Autodesk Inventor part; units mm, degrees
ref_plane "Work Plane2" through (0, 1, 0) normal (0, -1, 0) x (1, 0, 0)
ref_plane "YZ Plane" through (0, 0, 0) normal (1, 0, 0) x (0, 1, 0)
ref_plane "XZ Plane" through (0, 0, 0) normal (0, 1, 0) x (-1, 0, 0)
sketch "Sketch1" plane through (0, 0, 0) normal (0, 1, 0) x (-1, 0, 0)
  line L0 (0, 0) -> (20, 0)
  line L1 (20, 0) -> (20, -2)
  line L2 (20, -2) -> (0, -2)
  line L3 (0, -2) -> (0, 0)
  dimension "d0" = 20
  dimension "d1" = 2
extrude "Extrusion1" add sketch "Sketch1" along normal blind 2
sketch "Sketch2" plane through (0, 2, 0) normal (0, 1, 0) x (1, 0, 0)
  line L0 (0, 2) -> (-20, 2)
  line L1 (0, 2) -> (0, 4)
  line L2 (0, 4) -> (2, 4)
  line L3 (2, 4) -> (2, -2)
  line L4 (2, -2) -> (0, -2)
  line L5 (0, 0) -> (0, 2)
  line L6 (0, -2) -> (0, 0)
  dimension "d4" = 2
  dimension "d5" = 2
  dimension "d6" = 6
extrude "Extrusion2" add sketch "Sketch2" against normal blind 2
sketch "Sketch3" plane through (0, 2, 0) normal (0, 1, 0) x (1, 0, 0)
  line L0 (0, 0) -> (0, -2)
  line L1 (0, -2) -> (0, -1)
  line L2 (2, 4) -> (2, -2)
  line L3 (2, -2) -> (2, -0.5)
  line L4 (2, -0.5) -> (1, -0.5)
  circle A0 centre (1, -0.5) radius 0.5
  line L5 (2, 1) -> (1.5, 1)
  circle A1 centre (1, 2.5) radius 0.5
  dimension "d9" = 1.5
  dimension "d10" = 1
  dimension "d11" = 1
extrude "Extrusion3" cut sketch "Sketch3" against normal blind 2
sketch "Sketch4" plane through (0, 2, -4) normal (-1, 0, 0) x (0, 0, 1)
  line L0 (2, 0) -> (4, 0)
  line L1 (3, 0) -> (3, -2)
  line L2 (2, -2) -> (4, -2)
  circle A0 centre (3, -1) radius 1
  line L3 (2, -2) -> (2, 0)
  circle A1 centre (3, -1) radius 1.4142
extrude "Extrusion4" cut sketch "Sketch4" along normal blind 100 contours L0 A0 L3 | L3 A1 | L0 A1 L2 A0 | A0 L2 L3
ref_plane "Work Plane1" through (-14, 1, -1) normal (-1, 0, 0) x (0, 0, 1)
sketch "Sketch5" plane through (-14, 1, -1) normal (-1, 0, 0) x (0, 0, 1)
  circle A0 centre (0, 0) radius 5
  point P0 (1, -1)
  dimension "d17" = 10
extrude "Extrusion5" add sketch "Sketch5" along normal mid plane 1
sketch "Sketch6" plane through (-20, 1, -1) normal (-1, 0, 0) x (0, 0, 1)
  circle A0 centre (0, 0) radius 5
  point P0 (1, -1)
extrude "Extrusion6" cut sketch "Sketch6" against normal blind 5.5
sketch "Sketch7" plane through (-13.5, 1, -1) normal (1, 0, 0) x (0, 0, -1)
  circle A0 centre (0, 0) radius 5
  circle A1 centre (0, 0) radius 5
  point P0 (-1, -1)
extrude "Extrusion7" add sketch "Sketch7" along normal blind 13.5
sketch "Sketch8" plane through (0, 0, 0) normal (0, -1, 0) x (1, 0, 0)
  line L0 (2, -4) -> (-1, -4)
  line L1 (-1, -4) -> (-1, -6.7389)
  line L2 (-1, -6.7389) -> (2, -6.7389)
  line L3 (2, -6.7389) -> (2, -4)
  line L4 (2, -4) -> (2, 2)
  line L5 (2, 2) -> (-1, 2)
  line L6 (-1, 2) -> (-1, 5.2785)
  line L7 (-1, 5.2785) -> (2, 5.2785)
  line L8 (2, 5.2785) -> (2, 2)
  line L9 (2, 5.2785) -> (-1, 5.2785)
  line L10 (-1, 5.2785) -> (-1, -6.7389)
  line L11 (-1, -6.7389) -> (2, -6.7389)
  line L12 (2, -6.7389) -> (2, 5.2785)
  point P0 (0, 0)
  dimension "d24" = 3
  dimension "d25" = 3
extrude "Extrusion8" cut sketch "Sketch8" along normal blind 13.5
ref_plane "Work Plane2" through (0, 1, 0) normal (0, -1, 0) x (1, 0, 0)
mirror "Mirror1" about plane through (0, 1, 0) normal (0, -1, 0) of "Extrusion8"
properties part number "drive_shaft_v3"
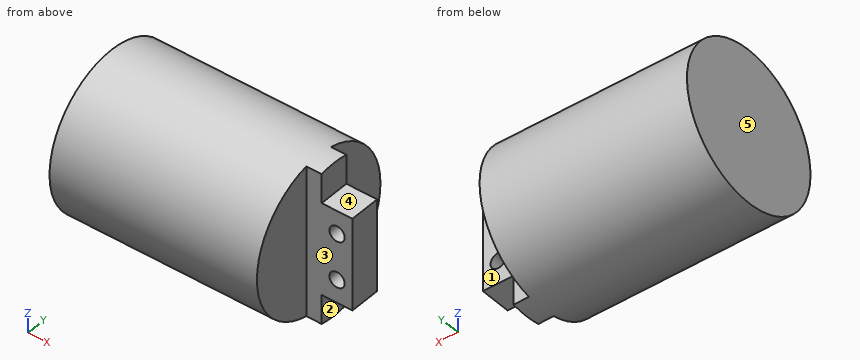
Input: part model. Units: mm. Frame: model coordinates. Face numbers are marked on the shaded views. A direction names the side the tool comes from. Coordinates: 2 decimals unless noted, no trailing zeros. Write each loop counter-clockwise with the first axis right and the second up, starting at its lowest first coordinate (ties: lowest second). Pieces come first, ordered by that corner, then holes.
1) Section D-D on z = -1. Output: boundary loops of the cut face in (x, y), and give its area (3 significant figures).
2) Material intervals for line 1 along Z through (x, y) = (1, 0.4); line 2 along X through (y, z) = (0.55, -2.5); line 3 along X through (y, z) = (-1.5, -2.25), sorted ascending.
3) Section B-B on y = 1. Output: boundary loops of the cut face in (x, z).
4) Pin query (flat end, axial travel): pin 1 Ø2.5 at (x, z) = (1, -3.5) entering from +Y; pin 2 Ø0.6 at (x, y) = (1, 1) entering from -Z; pin 3 Ø2 at (y, z) = (0.5, 2.5) entering from +X; pin 4 Ø1 at (x, y) = (-6, 4.5) entering from +Z. Return the tip coordinate at first contact, or that it passes through.
5) Section A-A on x = 1. Output: boundary loops of the cut face in (y, z).
6) Set-up query: the marked faces 1, 2, 3, 4 and 5. Return all of +Z, -Z, +X, -X, +Y, -Y with unobstructed straight access to the full face (end or side cutting, diameter ignored); none if empty.
7) Section C-C on z = 0.5. Output: boundary loops of the cut face in (x, y), and give its area (3 significant figures).
Check result:
1. outline: (-14.5, -4) - (-1, -4) - (-1, 0) - (2, 0) - (2, 2) - (-1, 2) - (-1, 6) - (-14.5, 6) - close
1. area: 141 mm2
2. line 1: z = -4 to -3, -2 to 0, 1 to 2
2. line 2: x = -14.5 to 0.5, 1.5 to 2
2. line 3: x = -14.5 to -1
3. outline: (-14.5, -6) - (0, -6) - (0, -4) - (2, -4) - (2, 2) - (0, 2) - (0, 4) - (-14.5, 4) - close; hole circle Ø1 at (1, -2.5); hole circle Ø1 at (1, 0.5)
4. pin 1: stops at y = 2
4. pin 2: stops at z = -4
4. pin 3: stops at x = 2
4. pin 4: stops at z = 3
5. outline: (0, -4) - (2, -4) - (2, -3) - (0, -3) - close; (0, -2) - (2, -2) - (2, 0) - (0, 0) - close; (0, 1) - (2, 1) - (2, 2) - (0, 2) - close
6. face 1: +Z, -Z, +X, +Y
6. face 2: -Z, +X, +Y, -Y
6. face 3: +Z, -Z, +X, -Y
6. face 4: +Z, +X, +Y, -Y
6. face 5: +Z, -Z, -X, +Y, -Y
7. outline: (-14.5, -3.77) - (-1, -3.77) - (-1, 0) - (0.5, 0) - (0.5, 2) - (-1, 2) - (-1, 5.77) - (-14.5, 5.77) - close; (1.5, 0) - (2, 0) - (2, 2) - (1.5, 2) - close
7. area: 133 mm2
